```python
from build123d import *

# Parameters (mm, degrees)
CROQUIS2_R                       = 1.65
CROQUIS2_R_2                     = 5
SALIENTE_EXTRUIR1_DEPTH          = 3.175
TALADRO_DE_MARGEN_PARA_M51_D     = 5.5
TALADRO_DE_MARGEN_PARA_M51_DEPTH = 6
TALADRO_DE_MARGEN_PARA_M51_TIP   = 1.652366702
REDONDEO1_R                      = 20


with BuildPart() as part:
    # Croquis2 → Saliente-Extruir1 (new body)
    with BuildSketch(Plane.XY.offset(64.203907482)):
        with BuildLine():
            Line((82.563009481, 31.349424269), (74.351031643, 25.577646382))
            Line((74.351031643, 25.577646382), (17.351031643, 25.577646382))
            ThreePointArc((17.351031643, 25.577646382), (6.351031643, 14.577646382), (17.351031643, 3.577646382))
            Line((17.351031643, 3.577646382), (74.351031643, 3.577646382))
            Line((74.351031643, 3.577646382), (82.563009481, -2.194131506))
            ThreePointArc((82.563009481, -2.194131506), (114.851031643, 14.577646382), (82.563009481, 31.349424269))
        make_face()
        with Locations((94.351031643, -0.922353618)):
            Circle(CROQUIS2_R, mode=Mode.SUBTRACT)
        with Locations((80.927637885, 6.827646382)):
            Circle(CROQUIS2_R, mode=Mode.SUBTRACT)
        with Locations((80.927637885, 22.327646382)):
            Circle(CROQUIS2_R, mode=Mode.SUBTRACT)
        with Locations((94.351031643, 30.077646382)):
            Circle(CROQUIS2_R, mode=Mode.SUBTRACT)
        with Locations((107.774425402, 22.327646382)):
            Circle(CROQUIS2_R, mode=Mode.SUBTRACT)
        with Locations((107.774425402, 6.827646382)):
            Circle(CROQUIS2_R, mode=Mode.SUBTRACT)
        with Locations(Location((17.351031643, 14.577646382, 0), (0, 0, 180))):
            Circle(CROQUIS2_R_2, mode=Mode.SUBTRACT)
        with BuildLine():
            Line((87.351031643, 21.177646382), (101.351031643, 21.177646382))
            ThreePointArc((101.351031643, 21.177646382), (107.951031643, 14.577646382), (101.351031643, 7.977646382))
            Line((101.351031643, 7.977646382), (87.351031643, 7.977646382))
            ThreePointArc((87.351031643, 7.977646382), (80.751031643, 14.577646382), (87.351031643, 21.177646382))
        make_face(mode=Mode.SUBTRACT)
    extrude(amount=SALIENTE_EXTRUIR1_DEPTH)

    # Taladro de margen para M51
    with Locations(Plane(origin=(0, 0, 64.203907482), x_dir=(-1, 0, 0), z_dir=(0, 0, -1))):
        with Locations((-65.351031643, 14.577646382), (-40.351031643, 14.577646382)):
            Hole(TALADRO_DE_MARGEN_PARA_M51_D / 2, depth=TALADRO_DE_MARGEN_PARA_M51_DEPTH)
            with Locations((0, 0, -(TALADRO_DE_MARGEN_PARA_M51_DEPTH + TALADRO_DE_MARGEN_PARA_M51_TIP / 2))):  # 118° drill point
                Cone(0, TALADRO_DE_MARGEN_PARA_M51_D / 2, TALADRO_DE_MARGEN_PARA_M51_TIP, mode=Mode.SUBTRACT)

    # Redondeo1
    redondeo1_edges = [part.edges().sort_by_distance(p)[0] for p in [
        (74.351031643, 3.577646382, 65.791407482),
        (74.351031643, 25.577646382, 65.791407482),
    ]]
    fillet(redondeo1_edges, radius=REDONDEO1_R)


solid = part.part
```
Design review of the part built by this model. Coordinates are the model's own, in mm. A direction names the side the tool comes from. Give positions to 0.01 mm unless a question says otherwise; leave off trailing zeros. Order: outer loops, then holes, each group sorted by start corner. A loop starts at its lowest first (then second) coordinate and runs counter-clockwise, first axis right, second up. Notation, with made-up numbers: (1, -33.75) -> (50, -33.75) arc R16 cw to (50, -22.75) -> close; hole circle Ø3 at (52, 39). An arc over 180 degrees is marked (long way). Write each question's results on one line, items separated by ' | '. Start each with the question number.
Q1. Add section B-B on z = 64.75. State how many separate pieces and enclosed holes the cut face has, and give its area (3 significant figures).
Q2. Machinability: for faces 5 (the cylindrical face through (107.95, 14.72, 65.77)), 6 (the cylindrical face through (6.354, 14.82, 65.769)), which of the approach directions +Z, -Z, +X, -X, +Y, -Y give a long, thin tool a straight path to every point of the face, cutting with its end or side? Answer none if there is none.
Q3. For pin 1 (10 mm diameter, centred on x = 48.5, y = 28, fed in from -Z); pin 2 (2.5 mm diameter, centred on x = 107.77, y = 22.33, fed in from +Z); pin 3 (1 mm diameter, centred on x = 40.5, z = 66, fed in from -Y); pin 4 (1.6 mm diameter, centred on x = 32.5, z = 66, fed in from +Y), all flat-tipped, find the tip position at first contact; note any pin that passes through.
Q4. Add section D-D on x = 71.5. Give the boundary of the cut face in (y, z).
Q5. Mouldability with a two-part tool opening along Y and no side actions: class faces 1 (the flat face through (42, 3.578, 66)), 2 (the flat face through (94, 21.178, 66)), 3 (the flat face through (43, 25.578, 66)), 4 (the flat face through (60, 15, 67.379)) as +Y half, -Y half, draft (parallel to the pull), parting line (faces both ways), or undercut.
Q6. Wall thickness on L1, parallel to X at y = 17, z = 67.1; L2, parallel to X at y = 19, z = 65.35; L3, parallel to X at y = 22, z = 66: over which ranges is each line inside the solid? List them lowest first. Write a range as from..to.
Q7. Add section A-A on x = 91. Give the boundary of the cut face in (y, z).
Q8. Add section C-C on x = 31.5. Give the boundary of the cut face in (y, z).
Found:
1) separate pieces: 1 | enclosed holes: 10 | area: 2,300 mm2
2) face 5: +Z, -Z | face 6: +Z, -Z, -X
3) pin 1: stops at z = 64.2 | pin 2: passes through | pin 3: stops at y = 3.58 | pin 4: stops at y = 25.58
4) outline: (3.27, 64.2) -> (25.88, 64.2) -> (25.88, 67.38) -> (3.27, 67.38) -> close
5) face 1: -Y half | face 2: undercut | face 3: +Y half | face 4: draft
6) L1: x = 6.62..12.98, 21.73..39.05, 41.65..64.05, 66.65..81.21, 107.49..114.71 | L2: x = 7.28..15.02, 19.68..82.45, 106.25..114.37 | L3: x = 9.23..79.31, 82.54..106.16, 109.39..113.46
7) outline: (-5.65, 64.2) -> (7.98, 64.2) -> (7.98, 67.38) -> (-5.65, 67.38) -> close; (21.18, 64.2) -> (34.8, 64.2) -> (34.8, 67.38) -> (21.18, 67.38) -> close
8) outline: (3.58, 64.2) -> (25.58, 64.2) -> (25.58, 67.38) -> (3.58, 67.38) -> close
